```python
from build123d import *

# Parameters (mm, degrees)
BOSS_EXTRUDE1_DEPTH = 25.4
CUT_EXTRUDE1_DEPTH  = 5.08
SKETCH3_OUTSIDE_W   = 13.788
SKETCH3_OUTSIDE_H   = 14.77
SKETCH3_OUTSIDE_R   = 3.175
CUT_EXTRUDE2_DEPTH  = 13.7


with BuildPart() as part:
    # Sketch1 → Boss-Extrude1 (new body)
    with BuildSketch(Plane.XY):
        Polygon((0, 3.666174209), (-3.175, 1.833087105), (-3.175, -1.833087105), (0, -3.666174209), (3.175, -1.833087105), (3.175, 1.833087105), align=None)
    extrude(amount=-BOSS_EXTRUDE1_DEPTH)

    # Sketch2 → Cut-Extrude1 (cut)
    with BuildSketch(Plane.XY):
        with BuildLine():
            Line((-1.303529881, -0.72898), (1.303529881, -0.72898))
            ThreePointArc((1.303529881, -0.72898), (0, 1.49352), (-1.303529881, -0.72898))
        make_face()
    extrude(amount=-CUT_EXTRUDE1_DEPTH, mode=Mode.SUBTRACT)

    # Sketch3 outside → Cut-Extrude2 (cut, through all)
    with BuildSketch(Plane.XY.offset(-12.7)):
        Rectangle(SKETCH3_OUTSIDE_W, SKETCH3_OUTSIDE_H)
        Circle(SKETCH3_OUTSIDE_R, mode=Mode.SUBTRACT)
    extrude(amount=-CUT_EXTRUDE2_DEPTH, mode=Mode.SUBTRACT)


solid = part.part
```
Here's how the part is built. I have some questions about the finished solid (model axes, mm). A direction names the side the tool comes from. Coordinates: 2 decimals unless noted, no trailing zeros. Write each loop counter-clockwise with the first axis right and the second up, starting at its lowest first coordinate (ties: lowest second). Pieces come first, ordered by that corner, then holes. Notation, with made-up numbers: (41, 89.25) - (73, 89.25) arc R10 ccw to (73, 95.25) - close; hole circle Ø9 at (20.5, 66.25). An arc over 180 degrees is marked (long way). One line per item, written item: value.
1) I need wall thicknesses on line 1 along X through (y, z) = (0, -2.95) (3 decimals); line 2 along Z through (x, y) = (2.75, -2); line 3 along Z through (x, y) = (-1.25, -0.5). Which ranges of each line are inside material? Lowest first, please.
Model answer:
line 1: x = -3.175 to -1.494, 1.494 to 3.175
line 2: z = -12.7 to 0
line 3: z = -25.4 to -5.08
2) Suppose I cut it at D-D on x = 1. Write out the boundary of the cut face in (y, z), and give its area (3 significant figures).
Model answer:
outline: (-3.09, -12.7) - (-3.01, -12.7) - (-3.01, -25.4) - (3.01, -25.4) - (3.01, -12.7) - (3.09, -12.7) - (3.09, 0) - (1.11, 0) - (1.11, -5.08) - (-0.73, -5.08) - (-0.73, 0) - (-3.09, 0) - close
area: 146 mm²
3) We'd pull the mould along Y, two halves only. Please class faces 5 (the flat face through (-2.9, -1.7, -12.7)), 6 (the flat face through (-1.61, -2.737, -6.261)), 7 (the cylindrical face through (0.043, 1.493, -2.504)): pulls with the +Y half, pulls with the -Y half, needs draft (parallel to the pull), parting line crosses it, or undercut.
Model answer:
face 5: needs draft
face 6: pulls with the -Y half
face 7: undercut
4) Suppose I cut it at C-C on z = -8. Write out the boundary of the cut face in (x, y) (3 decimals).
Model answer:
outline: (-3.175, -1.833) - (0, -3.666) - (3.175, -1.833) - (3.175, 1.833) - (0, 3.666) - (-3.175, 1.833) - close
5) Suppose I cut it at A-A on x = -2.5. Write out the boundary of the cut face in (y, z).
Model answer:
outline: (-2.22, -12.7) - (-1.96, -12.7) - (-1.96, -25.4) - (1.96, -25.4) - (1.96, -12.7) - (2.22, -12.7) - (2.22, 0) - (-2.22, 0) - close
6) On a 3-axis mill with a long thin cutter (end or side, diameter ignored), from which of +Z, -Z, +X, -X, +Y, -Y can I reach the whole of each face in a straight line? I mean faces 1 (the flat face through (0, 0, -5.08)), 2 (the flat face through (-2.9, 1.7, -12.7)), 3 (the flat face through (2.9, 1.7, -12.7)), 4 (the flat face through (-0.01, -3.34, -12.7)). Say none if no direction works.
Model answer:
face 1: +Z
face 2: -Z, -X, +Y
face 3: -Z, +X, +Y
face 4: -Z, -Y
7) I'm going to push a flat-ended pin straight in: P1, Ø1.5, axis at x = -1.5, z = -18.5, coming from the +Y side. Where does the tip first touch, or does it pass through?
Model answer:
P1: stops at y = 3.09
8) Suppose I cut it at B-B on y = -1. Write out the boundary of the cut face in (x, z) (3 decimals), and give its area (3 significant figures).
Model answer:
outline: (-3.175, -12.7) - (-3.013, -12.7) - (-3.013, -25.4) - (3.013, -25.4) - (3.013, -12.7) - (3.175, -12.7) - (3.175, 0) - (-3.175, 0) - close
area: 157 mm²
